```python
from build123d import *

# Parameters (mm, degrees)
F0_W     = 76.137118
F0_H     = 76.2
F1_DEPTH = 76.2
F4_D     = 25.4
F2_W     = 25.4
F2_H     = 25.4
F5_DEPTH = 12.7
F6_R     = 12.7
F7_DEPTH = 12.7


with BuildPart() as f1:
    # F0 (on Front) → F1 (new body)
    with BuildSketch(Plane.XZ):
        with Locations((38.068559, 38.1)):
            Rectangle(F0_W, F0_H)
    extrude(amount=F1_DEPTH)

    # F4 (through all)
    with Locations(Plane.XY.offset(76.2)):
        with Locations((35.253923, -38.1)):
            Hole(F4_D / 2)

    # F2 (on face) → F5 (join)
    with BuildSketch(Plane.XZ.offset(76.2)):
        with Locations((37.534562, 39.444917)):
            Rectangle(F2_W, F2_H)
    extrude(amount=F5_DEPTH)

    # F6 (on face) → F7 (join)
    with BuildSketch(Plane(origin=(0, 0, 0), x_dir=(-1, 0, 0), z_dir=(0, 1, 0))):
        with Locations((-38.1, 38.1)):
            Circle(F6_R)
    extrude(amount=F7_DEPTH)


solid = f1.part
```
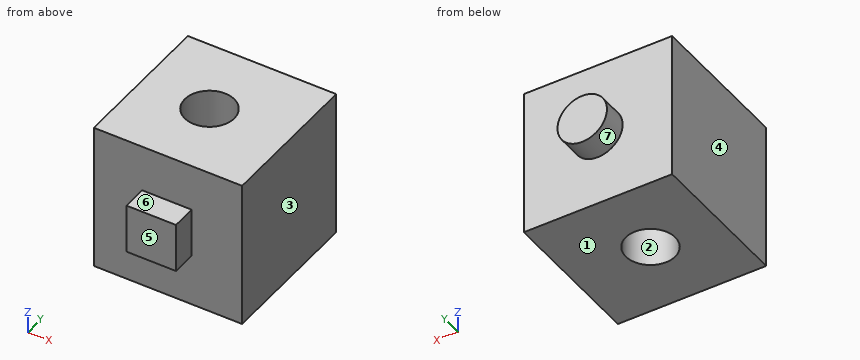
Model file for the job. Use its own axes, mm. Face numbers are marked on the shaded views. A direction names the side the tool comes from. Round coordinates to 2 decimals unless told otherwise and drop trailing zeros. Write each loop counter-clockwise with the first axis right and the second up, starting at its lowest first coordinate (ties: lowest second). Pieces come first, ordered by that corner, then holes. Notation, with made-up numbers: (-27, 64.25) - (10, 64.25) arc R9 ccw to (10, 79.25) - close; hole circle Ø10 at (-31.5, -25). An arc over 180 degrees is marked (long way). Use CSV: the item, a comma, the result in double quotes. Start each with the question number.
Item 1: Pin check, flat tips, straight feed: P1, Ø10, axis at x = 41, y = -83, coming from the -Z side; P2, Ø4, axis at x = 42.5, y = -85, coming from the +Z side; P3, Ø4, axis at y = -82.5, z = 38, coming from the -X side. Stop position of each tip, or through.
Item 2: Drill centre lines: L1, parallel to X at y = -78.5, z = 46; L2, parallel to Y at x = 68.5, z = 29; L3, parallel to Y at x = 25, z = 47.5. Where is each one in solid material? Low to high. Write a range as [from, to].
Item 3: Band-saw the part on B-B (y = -38.1). Write the cut outline in (x, z).
Item 4: Band-saw the part on A-A (z = 38.1). Write the cut outline in (x, y).
Item 5: Two-plate mould, pull along X, no slides. Class the marked faces 1, 2, 3 and 4: released by +X, released by -X, zero draft, split by the parting line, or undercut.
Item 6: Band-saw the part on D-D (x = 54). Write the cut outline in (y, z), and give its area (3 significant figures).
Item 7: Band-saw the part on C-C (x = 38.1). Write the cut outline in (y, z), and give its area (3 significant figures).
Item 8: Tool access for the marked faces 5, 6 and 7: list every direction of +Z, -Z, +X, -X, +Y, -Y with a clear straight run to the whole face (end or side of a thin tool).
Checked values:
1,P1,"stops at z = 26.74"
1,P2,"stops at z = 52.14"
1,P3,"stops at x = 24.83"
2,L1,"x = [24.83, 50.23]"
2,L2,"y = [-76.2, 0]"
2,L3,"y = [-88.9, -45.59], [-30.61, 0]"
3,outline,"(0, 0) - (22.55, 0) - (22.55, 76.2) - (0, 76.2) - close; (47.95, 0) - (76.14, 0) - (76.14, 76.2) - (47.95, 76.2) - close"
4,outline,"(0, -76.2) - (24.83, -76.2) - (24.83, -88.9) - (50.23, -88.9) - (50.23, -76.2) - (76.14, -76.2) - (76.14, 0) - (50.8, 0) - (50.8, 12.7) - (25.4, 12.7) - (25.4, 0) - (0, 0) - close; hole circle Ø25.4 at (35.25, -38.1)"
5,face 1,"zero draft"
5,face 2,"undercut"
5,face 3,"released by +X"
5,face 4,"released by -X"
6,outline,"(-76.2, 0) - (0, 0) - (0, 76.2) - (-76.2, 76.2) - close"
6,area,"5,810 mm²"
7,outline,"(-88.9, 26.74) - (-76.2, 26.74) - (-76.2, 0) - (-50.48, 0) - (-50.48, 76.2) - (-76.2, 76.2) - (-76.2, 52.14) - (-88.9, 52.14) - close; (-25.72, 0) - (0, 0) - (0, 25.4) - (12.7, 25.4) - (12.7, 50.8) - (0, 50.8) - (0, 76.2) - (-25.72, 76.2) - close"
7,area,"4,570 mm²"
8,face 5,"+Z, -Z, +X, -X, -Y"
8,face 6,"+Z, +X, -X, -Y"
8,face 7,"+Y"
